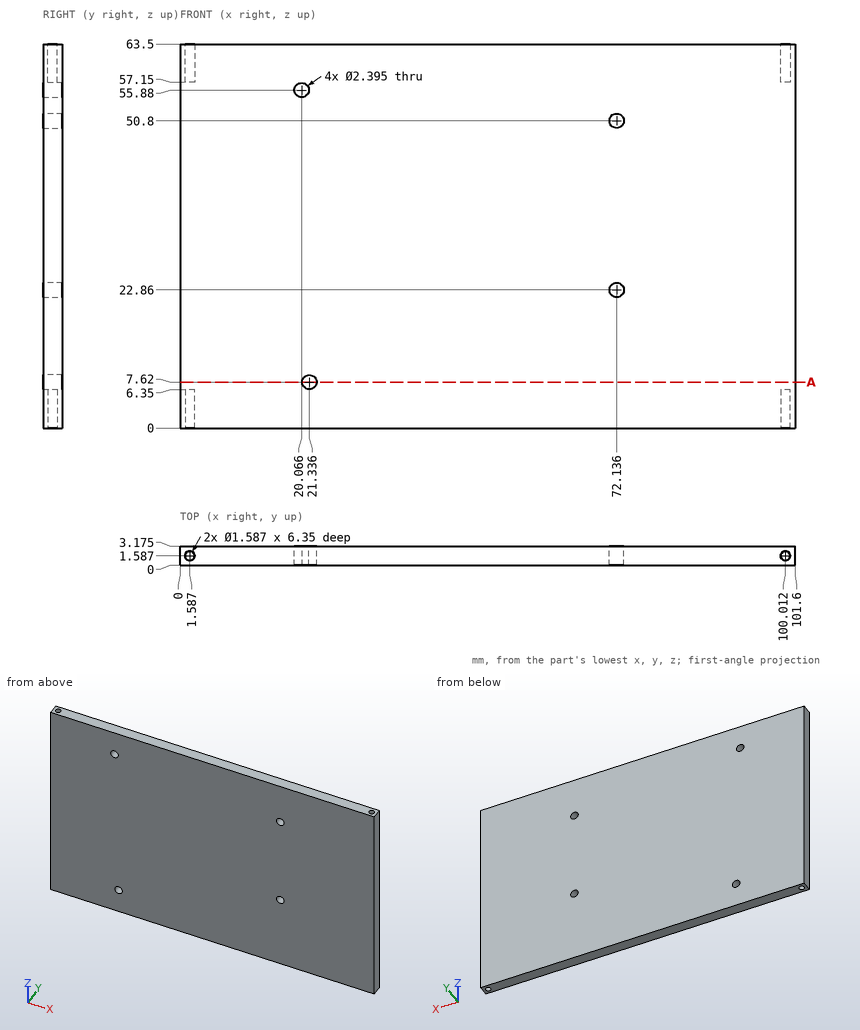
Print and shaded views of the part. All mm, measured from the part's lowest x, y and z. Coordinates: 2 decimals unless noted, no trailing zeros. Order: outer loops, then holes, each group sorted by start corner. A loop starts at its lowest first (then second) coordinate and runs counter-clockwise, first axis right, second up. Notation, with made-up numbers: (19, -23) - (72, -23) arc R20 cw to (72, 7) - close; hole circle Ø2 at (-9.5, 64.25). An arc over 180 degrees is marked (long way). Put each result on its own line as item: value.
1. Probe line 1 along X through (y, z) = (1.8, 55.88); line 2 along X through (y, z) = (1.8, 7.62). List the from-to ranges inside material, lowest first. Write a range as [from, to].
Answer sheet:
line 1: x = [0, 18.87], [21.26, 101.6]
line 2: x = [0, 20.14], [22.53, 101.6]
2. Saw through at A-A (z = 7.62). Write the cut outline in (x, y) (1 decimal).
Answer sheet:
outline: (0, 0) - (20.1, 0) - (20.1, 3.2) - (0, 3.2) - close; (22.5, 0) - (101.6, 0) - (101.6, 3.2) - (22.5, 3.2) - close
3. Drop flat-ended pins along their axis: P1, Ø0.5, axis at x = 100.5, y = 1.5, coming from the -Z side; P2, Ø1.9, axis at x = 72.136, z = 50.8, coming from the +Y side. Give the stop position or say it passes through.
Answer sheet:
P1: stops at z = 6.35
P2: passes through
